The figure shows three views and two pictorial views of one solid part (mm, origin at its lowest corner). Answer the questions. Coordinates: 2 decimals unless noted, no trailing zeros. Order: outer loops, then holes, each group sorted by start corner. A loop starts at its lowest first (then second) coordinate and runs counter-clockwise, first axis right, second up. Notation, with made-up numbers: M 72.25,31.5 L 99.25,31.5 A17 ccw 99.25,41.5 Z; hole C 68,23 d9. An arc over 180 degrees is marked long. Answer in a Markdown table with one row per item. Add a question column.
Item 1: The part is cut by section B-B (y = 3.6). Write down the section's boundary in (x, z), then the cut area to 3 significant figures.
Item 2: The part is cut by section A-A (z = 1.25). Write down the section's boundary in (x, y).
Item 3: Consider line 1 (X direction, y = 2.95, z = 0.5); line 2 (X direction, y = 4.55, z = 1); line 3 (Z direction, x = 142.5, y = 1.95). Determine where each line is inside the solid, lowest interval first. Write a range as from..to.
Item 4: The part is cut by section C-C (x = 140). Write down the section's boundary in (y, z).
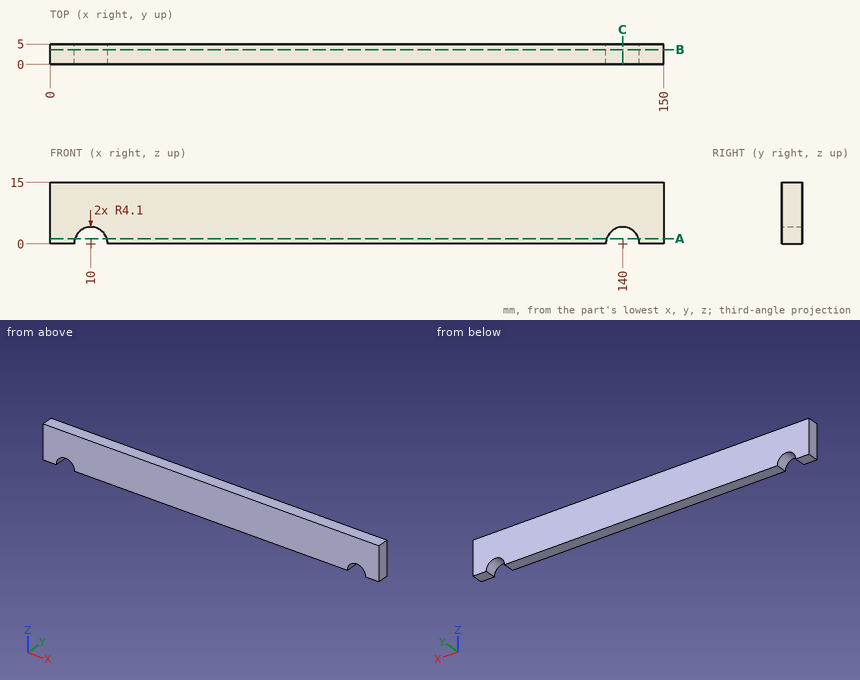
Reply:
| question | item | result |
|---|---|---|
| 1 | outline | M 0,0 L 5.9,0 A4.1 cw 14.1,0 L 135.9,0 A4.1 cw 144.1,0 L 150,0 L 150,15 L 0,15 Z |
| 1 | area | 2,200 mm2 |
| 2 | outline | M 0,0 L 6.1,0 L 6.1,5 L 0,5 Z; M 13.9,0 L 136.1,0 L 136.1,5 L 13.9,5 Z; M 143.9,0 L 150,0 L 150,5 L 143.9,5 Z |
| 3 | line 1 | x = 0..5.93, 14.07..135.93, 144.07..150 |
| 3 | line 2 | x = 0..6.02, 13.98..136.02, 143.98..150 |
| 3 | line 3 | z = 3.25..15 |
| 4 | outline | M 0,4.1 L 5,4.1 L 5,15 L 0,15 Z |
